Source: CAD feature listing. Evaluate the final solid. Frame: model axes, mm. Face numbers are marked on the shaded views. A direction names the side the tool comes from. Round coordinates to 2 decimals unless told otherwise and drop trailing zeros. Write each loop counter-clockwise with the first axis right and the second up, starting at its lowest first coordinate (ties: lowest second). Pieces come first, ordered by that corner, then holes. Notation, with made-up numbers: (68, -24) - (110, -24) arc R24 cw to (110, -6) - close; hole circle Ø10 at (10.5, -33). An arc over 180 degrees is marked (long way). Write item = value, one per line. Start each with the question number.
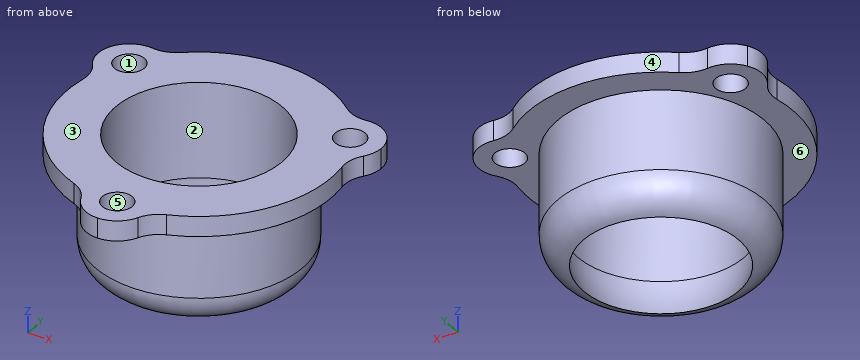
```python
from build123d import *

# Parameters (mm, degrees)
F1_W     = 8.89
F1_H     = 3.175
F3_R     = 2.38125
F4_DEPTH = 3.176
F7_DEPTH = 3.176
F8_R     = 5.08


# Not quite as in the source:
# - a fillet or chamfer that OpenCascade refuses, or shapes differently, is made with other operations: its cross-section is extruded or revolved along the edge and cut away or added


with BuildPart() as f2:
    # F1 (on Front) → F2 (revolve)
    with BuildSketch(Plane.XZ):
        with BuildLine():
            ThreePointArc((13.208, -11.9177163316), (13.0652297207, -14.7887805254), (12.3057501177, -17.5612494052))
            Line((12.3057501177, -17.5612494052), (16.383, -17.5612494052))
            Line((16.383, -17.5612494052), (16.383, 0))
            Line((16.383, 0), (16.383, 3.175))
            Line((16.383, 3.175), (13.208, 3.175))
            Line((13.208, 3.175), (13.208, -11.9177163316))
        make_face()
        with Locations((20.828, 1.5875)):
            Rectangle(F1_W, F1_H)
    revolve(axis=Axis((0, 0, -9.4681101426), (0, 0, 1)))

    # F3 (on face) → F4 (cut, through all)
    with BuildSketch(Plane(origin=(0, 0, 0), x_dir=(1, 0, 0), z_dir=(0, 0, -1))):
        with BuildLine():
            ThreePointArc((0, 17.93875), (1.6837980227, 18.6362019773), (2.38125, 20.32))
            ThreePointArc((2.38125, 20.32), (-1.6837980227, 22.0037980227), (0, 17.93875))
        make_face()
        with Locations((-17.5976362049, -10.16)):
            Circle(F3_R)
        with Locations((17.5976362049, -10.16)):
            Circle(F3_R)
    extrude(amount=-F4_DEPTH, mode=Mode.SUBTRACT)

    # F5: fillet of radius 5.08 on 1 edges, made by hand

    # F5_s1 → F5_t2 (revolve, cut)
    with BuildSketch(Plane.XZ):
        with BuildLine():
            ThreePointArc((12.3057501177, -17.5612494052), (15.2336723724, -15.7993073042), (16.383, -12.5811999876))
            Line((16.383, -12.5811999876), (16.383, -17.5612494052))
            Line((16.383, -17.5612494052), (12.3057501177, -17.5612494052))
        make_face()
    revolve(axis=Axis((0, 0, -17.5612494052), (0, 0, 1)), mode=Mode.SUBTRACT)

    # F6 (on face) → F7 (cut, through all)
    with BuildSketch(Plane(origin=(0, 0, 0), x_dir=(1, 0, 0), z_dir=(0, 0, -1))):
        with BuildLine():
            ThreePointArc((-4.952964542, 20.3387415379), (-3.495667473, 23.8289197652), (0, 25.273))
            ThreePointArc((0, 25.273), (-21.8870601005, 12.6364998776), (-21.8870598885, -12.6365002448))
            ThreePointArc((-21.8870598885, -12.6365002448), (-22.3842836342, -8.8871231844), (-20.0903491238, -5.8799776515))
            ThreePointArc((-20.0903491238, -5.8799776515), (-18.1286292594, 10.4665689829), (-4.952964542, 20.3387415379))
        make_face()
        with BuildLine():
            ThreePointArc((0, 25.273), (3.495667473, 23.8289197652), (4.952964542, 20.3387415379))
            ThreePointArc((4.952964542, 20.3387415379), (18.1286292594, 10.4665689829), (20.0903491238, -5.8799776515))
            ThreePointArc((20.0903491238, -5.8799776515), (21.8917377458, -7.6916197707), (22.5506362049, -10.16))
            ThreePointArc((22.5506362049, -10.16), (22.3818668231, -11.4419307281), (21.8870600322, -12.6364999959))
            ThreePointArc((21.8870600322, -12.6364999959), (24.4118434084, -6.5411337246), (25.273, 0))
            ThreePointArc((25.273, 0), (17.8707096809, 17.8707096809), (0, 25.273))
        make_face()
        with BuildLine():
            ThreePointArc((-15.1373845818, -14.4587638864), (-18.8886159884, -14.9417967542), (-21.8870598885, -12.6365002448))
            ThreePointArc((-21.8870598885, -12.6365002448), (1.437e-07, -25.273), (21.8870600322, -12.6364999959))
            ThreePointArc((21.8870600322, -12.6364999959), (18.8886161272, -14.9417967167), (15.1373845818, -14.4587638864))
            ThreePointArc((15.1373845818, -14.4587638864), (0, -20.9331379659), (-15.1373845818, -14.4587638864))
        make_face()
    extrude(amount=-F7_DEPTH, mode=Mode.SUBTRACT)

    # F8
    f8_edges = [f2.edges().sort_by_distance(p)[0] for p in [
        (-15.137385, 14.458764, 1.5875),
        (15.137385, 14.458764, 1.5875),
        (20.090349, 5.879978, 1.5875),
        (4.952965, -20.338742, 1.5875),
        (-4.952965, -20.338742, 1.5875),
        (-20.090349, 5.879978, 1.5875),
    ]]
    fillet(f8_edges, radius=F8_R)


solid = f2.part
```
(1) Reachability of the marked faces 5 and 6 from +Z, -Z, +X, -X, +Y, -Y: full face, straight path, thin tool, end or side. Return the list, or none.
(2) Section D-D (y = -17). Return the cut outline in (x, z) (3 decimals).
(3) Section B-B (z = -2.75). Return the cut outline in (x, y).
(4) Section A-A (y = 0). Return the cut outline in (x, z) (3 decimals), plus the area to 3 significant figures.
(5) Pull-direction query (Y, two-part tool) for the marked faces 1, 2, 3 and 4; classes: +Y half, -Y half, draft (parallel to the pull), parting line (faces both ways), or undercut.
(6) Section C-C (z = -13.5). Return the cut outline in (x, y), plus the area to 3 significant figures.
(7) Contact query for flat-ended pins moving along their axis: P1, Ø3, axis at x = -17.6, y = 10.16, coming from the -Z side; P2, Ø1, axis at x = 3, z = 0, coming from the -Y side; P3, Ø1, axis at x = -5.5, z = -7.5, coming from the -Y side; P4, Ø22.5, axis at x = 8, y = 3, coming from the -Z side. Output: stop coordinate, or through.
(8) Ray query, L1, parallel to Y at x = 0, z = -6.75; L2, parallel to Z at x = 7, y = -15 (3 decimals); L3, parallel to X at y = 2, z = -14. Return the intervals inside material, ascending. Write a range as from..to.
Solution:
q1.face_5 = +Z, -Z
q1.face_6 = -Z
q2.outline = (-12.215, 0) - (12.215, 0) - (12.215, 3.175) - (-12.215, 3.175) - close
q3.outline = circle Ø32.77 at (0, 0); hole circle Ø26.42 at (0, 0)
q4.outline = (-20.933, 0) - (-16.383, 0) - (-16.383, -12.581) arc R5.08 ccw to (-12.306, -17.561) arc R13.231 cw to (-13.208, -11.918) - (-13.208, 3.175) - (-20.933, 3.175) - close; (12.306, -17.561) arc R5.08 ccw to (16.383, -12.581) - (16.383, 0) - (20.933, 0) - (20.933, 3.175) - (13.208, 3.175) - (13.208, -11.918) arc R13.231 cw to start
q4.area = 153 mm^2
q5.face_1 = undercut
q5.face_2 = undercut
q5.face_3 = draft
q5.face_4 = +Y half
q6.outline = circle Ø32.6 at (0, 0); hole circle Ø26.41 at (0, 0)
q6.area = 287 mm^2
q7.P1 = through
q7.P2 = -24.6
q7.P3 = -15.6
q7.P4 = -17.56
q8.L1 = -16.38..-13.21, 13.21..16.38
q8.L2 = 0..3.175
q8.L3 = -16.06..-13.01, 13.01..16.06
